Part model, mm, in its own coordinate system. A direction names the side the tool comes from. Round coordinates to 2 decimals unless told otherwise and drop trailing zeros. Write each loop counter-clockwise with the first axis right and the second up, starting at its lowest first coordinate (ties: lowest second). Pieces come first, ordered by that corner, then holes. Notation, with made-up numbers: M 33.5,10.5 L 61.5,10.5 A15 ccw 61.5,38.5 Z; hole C -7.5,69 d1. An arc over 180 degrees is marked long. Answer as a JSON object with one key per item and string values. Group by question number.
1. Two-plate mould, pull along X, no slides. Class faces 1 (the face through (8, 5.902, 526)), 2 (the face through (21.292, -19, 526)), 3 (the face through (-1.009, -19, 526)): +X half, -X half, draft (parallel to the pull), parting line (faces both ways), or undercut.
2. Band-saw the part on C-C, the plane z = 923. Write the cut outline in (x, y).
3. Drill centre lines: line 1 (X direction, y = -23, z = 571.5); line 2 (Y direction, x = 0.5, z = 778); line 3 (Z direction, x = -3, y = -7.5). Where is each one in solid material? Low to high. Write a range as from..to.
4. Band-saw the part on A-A, the plane y = -16.5. Write the cut outline in (x, z).
5. Band-saw the part on B-B, the plane x = 10.5. Write the cut outline in (y, z).
6. Which spindle directions (+Z, -Z, +X, -X, +Y, -Y) get a long thin tool onto all of the face, cutting with end or side? Do faces 4 (the face through (9, 2.804, 526)), 5 (the face through (19, -21.26, 1064.51)). Say none if no direction does.
7. Drop a flat-ended pin along its axis: pin 1 (5 mm diameter, centred on x = 18, y = -1.5, fed in from -Z). Give the stop position or say it passes through.
Autodesk Inventor part; units mm, degrees
ref_plane "YZ Plane" through (0, 0, 0) normal (1, 0, 0) x (0, 1, 0)
ref_plane "XZ Plane" through (0, 0, 0) normal (0, 1, 0) x (-1, 0, 0)
ref_plane "XY Plane" through (0, 0, 0) normal (0, 0, 1) x (1, 0, 0)
sketch "Sketch2" plane through (0, 0, 0) normal (0, 0, 1) x (1, 0, 0)
  line L0 (-4.1078, 5.9023) -> (21.2922, 5.9023)
  line L1 (21.2922, 5.9023) -> (21.2922, -44.8977)
  line L2 (21.2922, -44.8977) -> (-4.1078, -44.8977)
  line L3 (-4.1078, -44.8977) -> (-4.1078, 5.9023)
  line L4 (18.1934, 2.8035) -> (-1.009, 2.8035)
  line L5 (-1.009, 2.8035) -> (-1.009, -41.7989)
  line L6 (-1.009, -41.7989) -> (18.1934, -41.7989)
  line L7 (18.1934, -41.7989) -> (18.1934, 2.8035)
  point P0 (0, 0)
  dimension "d0" = 25.4
  dimension "d1" = 50.8
  dimension "d2" = 3.0988
extrude "Extrusion1" add sketch "Sketch2" along normal blind 1066.8
sketch "Sketch5" plane through (0, 0, 1066.8) normal (0, 0, 1) x (1, 0, 0)
  point P0 (0, 0)
sketch "Sketch6" plane through (-4.1078, 5.9023, 0) normal (0, 1, 0) x (1, 0, 0)
  line L0 (25.4, 0) -> (-1.2066, -26.6066)
  line L1 (0, 0) -> (0, -1066.8)
  line L2 (0, -25.4) -> (0, 0)
  line L3 (0, 0) -> (25.4, 0)
  line L4 (0, -1066.8) -> (25.4, -1066.8)
  line L5 (25.4, -1066.8) -> (-7.0638, -1034.3362)
  line L6 (25.4, -1066.8) -> (71.3108, -1066.8) construction
  line L7 (0, -1041.4) -> (0, -1066.8)
  line L8 (0, -1066.8) -> (25.4, -1066.8)
  point P0 (4.1078, 0)
  dimension "d11" = 135
extrude "Extrusion2" cut sketch "Sketch6" against normal blind 1066.8 contours L0 L1 L3
extrude "Extrusion3" cut sketch "Sketch6" against normal blind 1066.8 contours L5 L4 L1
properties part number "42in 2x1 boxbeam"
Worked answers:
{
 "1": {"face 1": "draft", "face 2": "+X half", "face 3": "undercut"},
 "2": {"outline": "M -4.11,-44.9 L 21.29,-44.9 L 21.29,5.9 L -4.11,5.9 Z; hole M -1.01,-41.8 L 18.19,-41.8 L 18.19,2.8 L -1.01,2.8 Z"},
 "3": {"line 1": "x = -4.11..-1.01, 18.19..21.29", "line 2": "y = -44.9..-41.8, 2.8..5.9", "line 3": "z = 24.29..1042.51"},
 "4": {"outline": "M -4.11,25.4 L -1.01,22.3 L -1.01,1044.5 L -4.11,1041.4 Z; M 18.19,3.1 L 21.29,0 L 21.29,1066.8 L 18.19,1063.7 Z"},
 "5": {"outline": "M -44.9,10.79 L -41.8,10.79 L -41.8,1056.01 L -44.9,1056.01 Z; M 2.8,10.79 L 5.9,10.79 L 5.9,1056.01 L 2.8,1056.01 Z"},
 "6": {"face 4": "+Z, -Z", "face 5": "+Z, -X, +Y, -Y"},
 "7": {"pin 1": "stops at z = 0.79"}
}
